Part print with two shaded views. Sizes in mm from the minimum x, y, z corner. A direction names the side the tool comes from. Give positions to 0.01 mm unless a question says otherwise; leave off trailing zeros. Order: outer loops, then holes, each group sorted by start corner. A loop starts at its lowest first (then second) coordinate and runs counter-clockwise, first axis right, second up. Notation, with made-up numbers: M 65.5,13 L 120.5,13 A18 cw 120.5,21 Z; hole C 87.25,-28.75 d7. An arc over 180 degrees is marked long. Return JSON: item names as keys, results as strings. Group by question number.
1. Slice it at B-B on x = 684. List the corners of the cut face in (y, z), then the cut area to 3 significant figures.
2. Wall check: probe 1 along Y at (x, z) = (823, 165); probe 2 along X at (y, z) = (61, 496). Give the ranges that are in metal, low to high. Write a range as [from, to].
3. 3-axis set-ups, long thin cutter, end or side, ignore diameter. For the marked faces 1 and 2: which of +Z, -Z, +X, -X, +Y, -Y reach the whole face in a straight line?
4. Slice it at C-C on y = 101. List the corners of the cut face in (x, z).
5. Slice it at A-A on z = 156. List the corners of the cut face in (x, y).
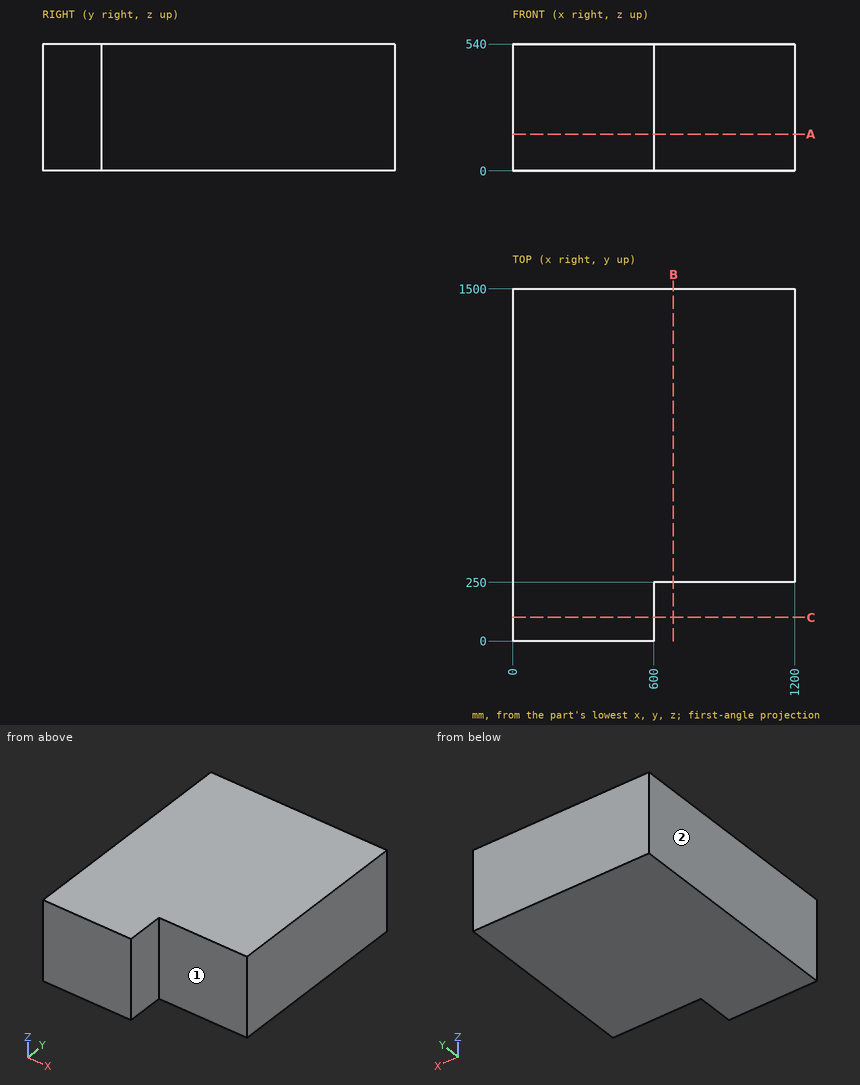
Result:
{
 "1": {"outline": "M 250,0 L 1500,0 L 1500,540 L 250,540 Z", "area": "675,000 mm2"},
 "2": {"probe 1": "y = [250, 1500]", "probe 2": "x = [0, 600]"},
 "3": {"face 1": "+Z, -Z, +X, -Y", "face 2": "+Z, -Z, -X, +Y, -Y"},
 "4": {"outline": "M 0,0 L 600,0 L 600,540 L 0,540 Z"},
 "5": {"outline": "M 0,0 L 600,0 L 600,250 L 1200,250 L 1200,1500 L 0,1500 Z"}
}
